Can you work these out from the model? Positions are in its coordinate system, mm. A direction names the side the tool comes from. Give positions to 0.01 mm unless a question says otherwise; leave off trailing zeros. Loops run counter-clockwise (first coordinate to the right, second up) from the corner with the lowest first, then second, coordinate; pieces in that order, holes last. Notation, with made-up numbers: (61, 38) -> (91, 38) arc R13 ccw to (91, 52) -> close; hole circle Ø4 at (30, 29). An arc over 180 degrees is marked (long way). One line per question, with ' | ' between items.
from build123d import *

# Parameters (mm, degrees)
F1_DEPTH     = 63.5
F0_W         = 25.4
F0_H         = 19.05
F0_H_2       = 4.7752
F0_H_3       = 4.7498
F2_DEPTH     = 25.4
F3_DEPTH     = 3.175
F5_T1_DEPTH  = 88.9
F5_T4_ANGLE  = 180
F6_T         = 2.54
F6_T3_DEPTH  = 24.13
F6_T5_DEPTH  = 27.305
F6_T7_DEPTH  = 68.58
F6_T9_DEPTH  = 27.305
F6_T11_DEPTH = 22.5552
F6_T13_DEPTH = 55.7790871697
F6_T15_DEPTH = 34.6589952471
F6_T18_ANGLE = 86.7817435726
F6_T20_ANGLE = 86.7817435726


# Not quite as in the source:
# - a fillet or chamfer that OpenCascade refuses, or shapes differently, is made with other operations: its cross-section is extruded or revolved along the edge and cut away or added
# - a shell that OpenCascade refuses in one call is made with other operations: the cavity is built on its own and cut out


with BuildPart() as f1:
    # F0 (on Front) → F1 (new body, symmetric)
    with BuildSketch(Plane.XZ):
        Polygon((41.275, -9.525), (41.275, 9.525), (22.225, 9.525), (-41.275, 9.525), (-41.275, -9.525), align=None)
    extrude(amount=F1_DEPTH, both=True)

    # F0 (on Front) → F2 (join, symmetric)
    with BuildSketch(Plane.XZ):
        with BuildLine():
            Line((22.225, 9.525), (41.275, 9.525))
            Line((41.275, 9.525), (41.275, 27.0002))
            ThreePointArc((41.275, 27.0002), (45.9246798487, 38.2255201513), (57.15, 42.8752))
            Line((57.15, 42.8752), (60.325, 42.8752))
            Line((60.325, 42.8752), (60.325, 61.9252))
            Line((60.325, 61.9252), (57.15, 61.9252))
            add(Edge.make_bspline(
                [(55.1893230691, 61.8701207193), (55.8379631981, 61.8888818572), (56.4915059272, 61.9072303668), (57.15, 61.9252)],
                knots=[110.4053566359, 110.4053566359, 110.4053566359, 110.4053566359, 111.5045361635, 111.5045361635, 111.5045361635, 111.5045361635], degree=3))
            ThreePointArc((55.1893230691, 61.8701207193), (31.7705568736, 50.9926882326), (22.225, 27.0002))
            Line((22.225, 27.0002), (22.225, 9.525))
        make_face()
        with Locations((73.025, 52.4002)):
            Rectangle(F0_W, F0_H)
        with Locations((73.025, 40.4876)):
            Rectangle(F0_W, F0_H_2)
        with Locations((73.025, 64.3001)):
            Rectangle(F0_W, F0_H_3)
    extrude(amount=F2_DEPTH, both=True)

    # F0 (on Front) → F3 (join, symmetric)
    with BuildSketch(Plane.XZ):
        with BuildLine():
            Line((-41.275, 9.525), (22.225, 9.525))
            Line((22.225, 9.525), (22.225, 27.0002))
            ThreePointArc((22.225, 27.0002), (31.7705568736, 50.9926882326), (55.1893230691, 61.8701207193))
            add(Edge.make_bspline(
                [(-41.275, 9.525), (-25.6521962788, 53.9382967597), (-9.9623131958, 59.9856877717), (55.1893230691, 61.8701207193)],
                knots=[0, 0, 0, 0, 110.4053566359, 110.4053566359, 110.4053566359, 110.4053566359], degree=3))
        make_face()
    extrude(amount=F3_DEPTH, both=True)

    # F0 (on Front) → F4 (revolve)
    with BuildSketch(Plane.XZ):
        Polygon((85.725, 61.9252), (85.725, 42.8752), (85.725, 38.1), (111.125, 38.1), (111.125, 66.675), (85.725, 66.675), align=None)
    revolve(axis=Axis((85.725, 0, 52.3875), (0, 0, 1)))

    # F5: fillet of radius 25.4 on 1 edges, made by hand

    # F5_s2 → F5_t1 (cut)
    with BuildSketch(Plane.YZ.offset(-3.175)):
        with BuildLine():
            ThreePointArc((0, 66.675), (17.9605122421, 59.2355122421), (25.4, 41.275))
            Line((25.4, 41.275), (25.4, 66.675))
            Line((25.4, 66.675), (0, 66.675))
        make_face()
        with BuildLine():
            ThreePointArc((0, 66.675), (-17.9605122421, 59.2355122421), (-25.4, 41.275))
            Line((-25.4, 41.275), (-25.4, 66.675))
            Line((-25.4, 66.675), (0, 66.675))
        make_face()
    extrude(amount=F5_T1_DEPTH, mode=Mode.SUBTRACT)

    # F5_s3 → F5_t4 (revolve, cut)
    with BuildSketch(Plane.YZ.offset(85.725)):
        with BuildLine():
            ThreePointArc((0, 66.675), (17.9605122421, 59.2355122421), (25.4, 41.275))
            Line((25.4, 41.275), (25.4, 66.675))
            Line((25.4, 66.675), (0, 66.675))
        make_face()
    revolve(axis=Axis((85.725, 0, 66.675), (0, 0, -1)), revolution_arc=F5_T4_ANGLE, mode=Mode.SUBTRACT)

    # F6: shell of thickness 2.54, made by hand


with BuildPart() as f6_core1:
    # F6_t2: copy of F1
    add(f1.part)

    # the walls: a layer under each face that stays
    f6_faces = [f6_core1.faces().sort_by_distance(p)[0] for p in [
        (41.275, 0, 8.7376),
        (0, 63.5, 0),
        (0, 33.3375, 9.525),
        (36.214543408, 25.4, 25.4),
        (45.9246798487, 0, 38.2255201513),
        (36.214543408, -25.4, 25.4),
        (0, -33.3375, 9.525),
        (0, -63.5, 0),
        (-41.275, 0, 0),
        (22.225, 14.2875, 18.2626),
        (6.9571615345, 3.175, 35.6975603597),
        (31.7705568736, 14.2875, 50.9926882326),
        (55.5002346295, 17.9605122421, 59.2355122421),
        (55.5002346295, -17.9605122421, 59.2355122421),
        (58.7375, 0, 42.8752),
        (31.7705568736, -14.2875, 50.9926882326),
        (22.225, -14.2875, 18.2626),
        (6.9571615345, -3.175, 35.6975603597),
        (-11.6161506693, 1.5875, 51.6458842892),
        (-11.6161506693, -1.5875, 51.6458842892),
        (56.1659663056, 7.4330512334, 61.8979571739),
        (60.325, 0, 64.3001),
        (58.7375, 0, 61.9252),
        (60.325, 0, 40.4876),
        (73.025, 25.4, 39.6875),
        (103.6855122422, -1e-10, 59.2355122421),
        (56.1659663056, -7.4330512334, 61.8979571739),
        (73.025, -25.4, 39.6875),
        (85.725, 0, 38.1),
        (111.125, 0, 39.6875),
    ]]
    thicken(f6_faces, amount=-F6_T, mode=Mode.SUBTRACT)

    # F6_s4 → F6_t3 (cut)
    with BuildSketch(Plane.YZ.offset(19.685)):
        Polygon((25.4254, 9.5504), (25.4, 6.985), (22.86, 6.985), (22.86, 9.525), align=None)
        Polygon((-25.4254, 9.5504), (-22.86, 9.525), (-22.86, 6.985), (-25.4, 6.985), align=None)
    extrude(amount=F6_T3_DEPTH, mode=Mode.SUBTRACT)

    # F6_s6 → F6_t5 (cut)
    with BuildSketch(Plane.XZ.offset(-27.94)):
        Polygon((22.1996, 9.5504), (22.225, 6.985), (24.765, 6.985), (24.765, 9.525), align=None)
    extrude(amount=F6_T5_DEPTH, mode=Mode.SUBTRACT)

    # F6_s8 → F6_t7 (cut)
    with BuildSketch(Plane.YZ.offset(-43.815)):
        Polygon((3.2004, 9.5504), (3.175, 6.985), (0.635, 6.985), (0.635, 9.525), align=None)
        Polygon((-3.2004, 9.5504), (-3.175, 6.985), (-0.635, 6.985), (-0.635, 9.525), align=None)
    extrude(amount=F6_T7_DEPTH, mode=Mode.SUBTRACT)

    # F6_s10 → F6_t9 (cut)
    with BuildSketch(Plane.XZ.offset(0.635)):
        Polygon((22.1996, 9.5504), (22.225, 6.985), (24.765, 6.985), (24.765, 9.525), align=None)
    extrude(amount=F6_T9_DEPTH, mode=Mode.SUBTRACT)

    # F6_s12 → F6_t11 (cut)
    with BuildSketch(Plane.XY.offset(6.985)):
        Polygon((22.1996, 3.2004), (24.765, 3.175), (24.765, 0.635), (22.225, 0.635), align=None)
        Polygon((22.1996, -3.2004), (24.765, -3.175), (24.765, -0.635), (22.225, -0.635), align=None)
    extrude(amount=F6_T11_DEPTH, mode=Mode.SUBTRACT)

    # F6_s14 → F6_t13 (cut)
    with BuildSketch(Plane.XZ.offset(-27.8895435848)):
        Polygon((60.2996, 42.8498), (60.325, 45.4152), (62.865, 45.4152), (62.865, 42.8752), align=None)
    extrude(amount=F6_T13_DEPTH, mode=Mode.SUBTRACT)

    # F6_s16 → F6_t15 (cut)
    with BuildSketch(Plane.XZ.offset(-17.3294976236)):
        Polygon((60.2996, 61.9506), (62.865, 61.9252), (62.865, 59.3852), (60.325, 59.3852), align=None)
    extrude(amount=F6_T15_DEPTH, mode=Mode.SUBTRACT)

    # F6_s17 → F6_t18 (revolve, cut)
    with BuildSketch(Plane.XY.offset(27.0002)):
        Polygon((22.1996, 3.2004), (22.225, 0.635), (24.765, 0.635), (24.765, 3.175), align=None)
    revolve(axis=Axis((57.15, 3.175, 27.0002), (0, 1, 0)), revolution_arc=F6_T18_ANGLE, mode=Mode.SUBTRACT)

    # F6_s19 → F6_t20 (revolve, cut)
    with BuildSketch(Plane.XY.offset(27.0002)):
        Polygon((22.1996, -3.2004), (24.765, -3.175), (24.765, -0.635), (22.225, -0.635), align=None)
    revolve(axis=Axis((57.15, -3.175, 27.0002), (0, 1, 0)), revolution_arc=F6_T20_ANGLE, mode=Mode.SUBTRACT)


with BuildPart() as f1_1:
    add(f1.part)

    # what is left inside the walls is the cavity
    f6_cavity = [f6_core1.part.solids().sort_by_distance(p)[0] for p in [
        (0, 20.32, -9.4996),
    ]]
    add(f6_cavity, mode=Mode.SUBTRACT)


solid = f1_1.part
Q1. On a 3-axis mill with a long thin cutter (end or side, diameter ignored), from which of +Z, -Z, +X, -X, +Y, -Y can I reach the whole of each face in a straight line? I mean faces 5 (the face through (45.8, -0.4, 38.1)), 6 (the face through (-4, -3.175, 36)), 7 (the face through (108.58, -0.5, 40.96)), 8 (the face through (22.225, 14, 18)). Say none if no direction works.
Entries:
face 5: -Z, +Y, -Y | face 6: +Z, -X, -Y | face 7: none | face 8: +Z, -X, +Y
Q2. If we section it at B-B (x = 94): Write out the boundary of the cut face in (y, z) (1 decimal), plus the area to 3 significant figures.
Entries:
outline: (-24, 38.1) -> (24, 38.1) -> (24, 41.3) arc R24 ccw to (-24, 41.3) -> close; hole (-21.3, 40.6) -> (21.3, 40.6) -> (21.3, 41.3) arc R21.3 ccw to (-21.3, 41.3) -> close | area: 318 mm²
Q3. If we mould it in two halves opening along X, with no side actions, what happens to faces 1 (the face through (-2, 0.635, 34)), 2 (the face through (60.325, 0, 64)), 3 (the face through (43.99, -0.32, 39.88)), 4 (the face through (111.12, -0.56, 39.71))? For each: pulls with the +X half, pulls with the -X half, needs draft (parallel to the pull), parting line crosses it, or undercut.
Entries:
face 1: undercut | face 2: pulls with the -X half | face 3: undercut | face 4: pulls with the +X half
Q4. If we section it at A-A (y = -41.5): Write out the boundary of the cut face in (x, z) (3 decimals), plus the area to 3 significant figures.
Entries:
outline: (-41.275, -9.525) -> (-38.735, -9.525) -> (-38.735, 6.985) -> (38.735, 6.985) -> (38.735, -9.525) -> (41.275, -9.525) -> (41.275, 9.525) -> (-41.275, 9.525) -> close | area: 294 mm²
Q5. For pin 1 Ø15 at (x, y) = (78, -2) entering from -Z; pin 2 Ø8.5 at (y, z) = (-16.5, 19) entering from -X (3 decimals); pin 3 Ø6 at (x, y) = (81.5, -26) entering from +Z; pin 4 Ø12 at (y, z) = (-34, 41.5) entering from +X, each with a flat end and sliding along its axis, tell me the tip position at first contact or that it passes through.
Entries:
pin 1: z = 38.1 | pin 2: x = 22.225 | pin 3: z = 52.05 | pin 4: through
Q6. If I drill on probe 1 along Y at (x, z) = (-24.5, 30) (3 decimals); probe 2 along X at (y, z) = (17.5, 12.5) (3 decimals); probe 3 along Y at (x, z) = (41, 40), over which ranges is the centre line in solid material (lowest first)? Write a range as from..to.
Entries:
probe 1: -3.175..-0.635, 0.635..3.175 | probe 2: 22.225..24.765, 38.735..41.275 | probe 3: -25.4..-22.86, 22.86..25.4
